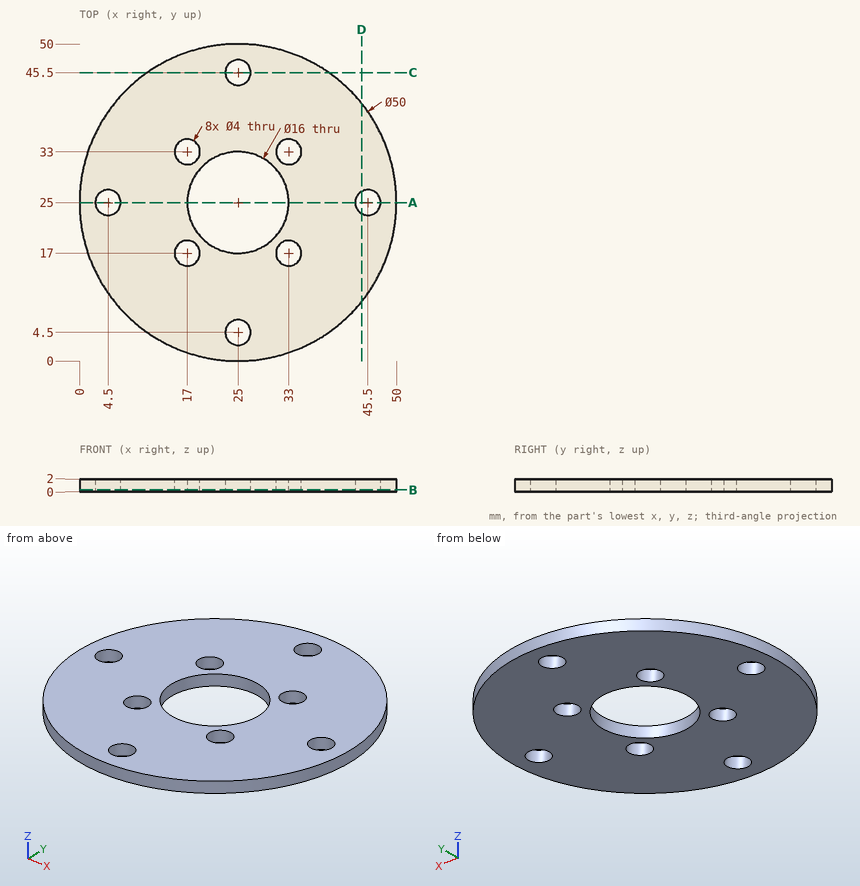
Design review of the part shown in the three views and the two pictorial views. Dimensions are in mm from the part's minimum x, y and z. Round coordinates to 2 decimals unless told otherwise and drop trailing zeros. Loops run counter-clockwise (first coordinate to the right, second up) from the corner with the lowest first, then second, coordinate; pieces in that order, holes last. Notation, with made-up numbers: (-26.75, -8) -> (-0.75, -8) arc R29 ccw to (-0.75, 16) -> close; hole circle Ø7 at (52.25, 79.25). An arc over 180 degrees is marked (long way). Return JSON: item names as keys, results as strings.
(1) Add section B-B on z = 0.3. State how many separate pieces and enclosed holes the cut face has, plus the area to 3 significant figures.
Solved:
{"separate pieces": "1", "enclosed holes": "9", "area": "1,660 mm2"}
(2) Add section C-C on y = 45.5. Write out the cut boundary in (x, z).
Solved:
{"outline": "(10.69, 0) -> (23, 0) -> (23, 2) -> (10.69, 2) -> close; (27, 0) -> (39.31, 0) -> (39.31, 2) -> (27, 2) -> close"}
(3) Add section A-A on y = 25. Write out the cut boundary in (x, z), plus the area to 3 significant figures.
Solved:
{"outline": "(0, 0) -> (2.5, 0) -> (2.5, 2) -> (0, 2) -> close; (6.5, 0) -> (17, 0) -> (17, 2) -> (6.5, 2) -> close; (33, 0) -> (43.5, 0) -> (43.5, 2) -> (33, 2) -> close; (47.5, 0) -> (50, 0) -> (50, 2) -> (47.5, 2) -> close", "area": "52.0 mm2"}
(4) For line 1 (Y direction, x = 25, z = 1.05); line 2 (X direction, y = 34, z = 1.9); line 3 (Y direction, x = 23.5, z = 1), list the stretches that pass through material, from the lowest coordinate up.
Solved:
{"line 1": "0 to 2.5, 6.5 to 17, 33 to 43.5, 47.5 to 50", "line 2": "1.68 to 15.27, 18.73 to 31.27, 34.73 to 48.32", "line 3": "0.05 to 3.18, 5.82 to 17.14, 32.86 to 44.18, 46.82 to 49.95"}
(5) For pin 1 (3 mm diameter, centred on x = 4.5, y = 25, fed in from -Z); pin 2 (6.5 mm diameter, centred on x = 17, y = 33, fed in from -Z), all flat-tipped, find the tip position at first contact; note any pin that passes through.
Solved:
{"pin 1": "through", "pin 2": "z = 0"}
(6) Add section D-D on x = 44.5. Write out the cut boundary in (y, z), plus the area to 3 significant figures.
Solved:
{"outline": "(9.36, 0) -> (23.27, 0) -> (23.27, 2) -> (9.36, 2) -> close; (26.73, 0) -> (40.64, 0) -> (40.64, 2) -> (26.73, 2) -> close", "area": "55.6 mm2"}
